The listing builds one solid part. Answer for the finished solid, in the listing's coordinates (mm). Face numbers are marked on the shaded views. Round coordinates to 2 decimals unless told otherwise and drop trailing zeros. Loops run counter-clockwise (first coordinate to the right, second up) from the corner with the lowest first, then second, coordinate; pieces in that order, holes last. Notation, with made-up numbers: (-19.5, 82.5) -> (-12.5, 82.5) arc R32 cw to (-12.5, 115.5) -> close; hole circle Ø5 at (23, -24.75). An arc over 180 degrees is marked (long way). Use a Markdown table: item, result. Add a question column.
Q1. Section A-A on x = -216 is taken. Give the vertices of the cut face in (y, z), then the cut area to 3 significant figures.
Q2. Section D-D on y = 95 is taken. Give the vertices of the cut face in (x, z).
Q3. Section B-B on y = 67 is taken. Give the vertices of the cut face in (x, z).
Q4. Given pin 1 Ø2 at (y, z) = (107.5, -4.5) entering from +X; pin 2 Ø2.5 at (y, z) = (0, 3.5) entering from +X; pin 3 Ø6 at (x, y) = (-211, 23.5) entering from -Z, each flat-ended and moving along its own axis, determine where each tip first touches the part or whether it passes through.
Q5. Section C-C on x = -155 is taken. Give the vertices of the cut face in (y, z).
Q6. For a pull along Y with two mould halves and no side action, classify the marked faces 1, 2 and 3 as released by +Y, released by -Y, zero draft, split by the parting line, or undercut.
Q7. Consider line 1 (Y direction, x = -203, z = 0.75); line 2 (X direction, y = 76, z = 4); line 3 (Y direction, x = -218.5, z = -1). Determine where each line is inside the solid, lowest interval first.
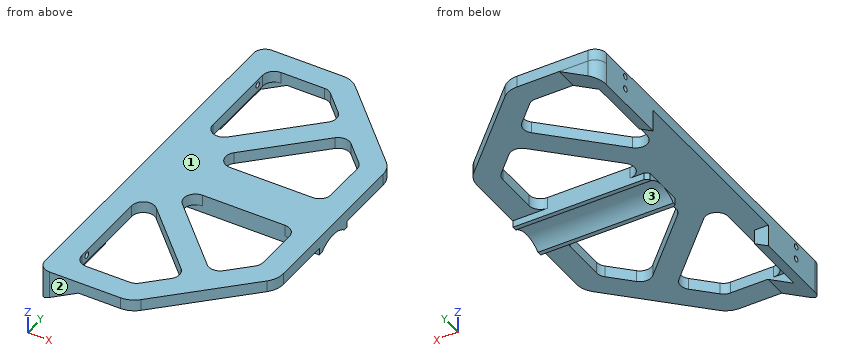
from build123d import *
from build123d.topology import SkipClean

# Parameters (mm, degrees)
RESSALTO_EXTRUS_O2_DEPTH   = 5
CORTE_EXTRUS_O1_DEPTH      = 5
FILETE1_R                  = 10
FILETE2_R                  = 5
ESBO_O7_W                  = 62.928932188
ESBO_O7_H                  = 19.982162149
RESSALTO_EXTRUS_O5_DEPTH   = 5
CORTE_EXTRUS_O2_DEPTH      = 66
FILETE3_R                  = 5
CORTE_EXTRUS_O5_DEPTH      = 35
RESSALTO_EXTRUS_O6_DEPTH   = 159.982162
ESBO_O12_W                 = 11.383352407
ESBO_O12_H                 = 139.982162149
CORTE_EXTRUS_O6_DEPTH      = 10
CORTE_EXTRUS_O7_DEPTH      = 10
CORTE_EXTRUS_O7_DEPTH_BACK = 146.645655307
ESBO_O14_R                 = 1.25
FILETE4_R                  = 5
ESBO_O16_W                 = 30.044355049
ESBO_O16_H                 = 82.897559044
CORTE_EXTRUS_O8_DEPTH      = 262.030945505


with BuildPart() as part:
    # Esboço1 → Ressalto-extrusão2 (new body)
    with BuildSketch(Plane.XY):
        Polygon((-148.870088073, 85.148606513), (-188.870088073, 125.148606513), (-228.870088073, 125.148606513), (-228.870088073, -34.833555636), (-188.870088073, -34.833555636), (-148.870088073, 5.166444364), align=None)
    extrude(amount=RESSALTO_EXTRUS_O2_DEPTH)

    # Esboço4 → Corte-extrusão1 (cut)
    with BuildSketch(Plane(origin=(0, 0, 0), x_dir=(-1, 0, 0), z_dir=(0, 0, -1))):
        Polygon((179.47668979, 101.613072607), (218.870088073, 62.219674325), (218.870088073, 115.148606513), (193.012223696, 115.148606513), align=None)
        Polygon((158.870088073, 55.148606513), (211.799020261, 55.148606513), (172.405621979, 94.542004796), (158.870088073, 81.00647089), align=None)
        Polygon((172.405621979, -4.226953918), (211.799020261, 35.166444364), (158.870088073, 35.166444364), (158.870088073, 9.308579988), align=None)
        Polygon((218.870088073, -24.833555636), (218.870088073, 28.095376552), (179.47668979, -11.29802173), (193.012223696, -24.833555636), align=None)
    extrude(amount=-CORTE_EXTRUS_O1_DEPTH, mode=Mode.SUBTRACT)

    # Filete1
    filete1_edges = [part.edges().sort_by_distance(p)[0] for p in [
        (-188.870088073, 125.148606513, 2.5),
        (-148.870088073, 85.148606513, 2.5),
        (-148.870088073, 5.166444364, 2.5),
        (-188.870088073, -34.833555636, 2.5),
    ]]
    fillet(filete1_edges, radius=FILETE1_R)

    # Filete2
    filete2_edges = [part.edges().sort_by_distance(p)[0] for p in [
        (-218.870088073, 115.148606513, 2.5),
        (-218.870088073, -24.833555636, 2.5),
    ]]
    fillet(filete2_edges, radius=FILETE2_R)

    # Esboço7 → Ressalto-extrusão5 (add)
    with BuildSketch(Plane(origin=(0, 0, 0), x_dir=(-1, 0, 0), z_dir=(0, 0, -1))):
        with Locations((180.334554167, 45.157525439)):
            Rectangle(ESBO_O7_W, ESBO_O7_H)
    extrude(amount=RESSALTO_EXTRUS_O5_DEPTH)

    # Esboço8 → Corte-extrusão2 (cut)
    with BuildSketch(Plane(origin=(-148.870088073, 0, 0), x_dir=(0, 0, -1), z_dir=(1, 0, 0))):
        with BuildLine():
            Line((3.009284908, 37.096966334), (3.009284908, 53.218084544))
            ThreePointArc((3.009284908, 53.218084544), (0, 45.157525439), (3.009284908, 37.096966334))
        make_face()
        with BuildLine():
            Line((5, 55.148606513), (3.009284908, 55.148606513))
            Line((3.009284908, 55.148606513), (3.009284908, 53.218084544))
            ThreePointArc((3.009284908, 53.218084544), (3.95384052, 54.192547406), (5, 55.057020375))
            Line((5, 55.057020375), (5, 55.148606513))
        make_face()
        with BuildLine():
            ThreePointArc((5, 55.057020375), (3.95384052, 54.192547406), (3.009284908, 53.218084544))
            Line((3.009284908, 53.218084544), (3.009284908, 37.096966334))
            ThreePointArc((3.009284908, 37.096966334), (3.95384052, 36.122503472), (5, 35.258030502))
            Line((5, 35.258030502), (5, 55.057020375))
        make_face()
        with BuildLine():
            ThreePointArc((5, 35.258030502), (3.95384052, 36.122503472), (3.009284908, 37.096966334))
            Line((3.009284908, 37.096966334), (3.009284908, 35.166444364))
            Line((3.009284908, 35.166444364), (5, 35.166444364))
            Line((5, 35.166444364), (5, 35.258030502))
        make_face()
    extrude(amount=-CORTE_EXTRUS_O2_DEPTH, mode=Mode.SUBTRACT)

    # Filete3
    filete3_edges = [part.edges().sort_by_distance(p)[0] for p in [
        (-218.870088073, 62.219674325, 2.5),
        (-211.799020261, 55.148606513, 2.5),
        (-211.799020261, 35.166444364, 2.5),
        (-218.870088073, 28.095376552, 2.5),
        (-193.012223696, -24.833555636, 2.5),
        (-179.47668979, -11.29802173, 2.5),
        (-172.405621979, -4.226953918, 2.5),
        (-158.870088073, 9.308579988, 2.5),
        (-158.870088073, 55.148606513, 2.5),
        (-179.47668979, 101.613072607, 2.5),
        (-193.012223696, 115.148606513, 2.5),
        (-158.870088073, 81.00647089, 2.5),
        (-172.405621979, 94.542004796, 2.5),
        (-158.870088073, 35.166444364, 2.5),
    ]]
    fillet(filete3_edges, radius=FILETE3_R)

    # Esboço9 → Corte-extrusão5 (cut)
    # profile 1 of 2: a face of its own
    with BuildSketch(Plane(origin=(0, 0, 0), x_dir=(-1, 0, 0), z_dir=(0, 0, -1))):
        with BuildLine():
            Line((148.870088073, 62.717943557), (158.870088073, 61.569782302))
            Line((158.870088073, 61.569782302), (158.870088073, 78.935403078))
            ThreePointArc((158.870088073, 78.935403078), (159.25069041, 80.84882024), (160.334554167, 82.470936984))
            Line((160.334554167, 82.470936984), (168.870088073, 91.00647089))
            ThreePointArc((168.870088073, 91.00647089), (172.405621979, 92.470936984), (175.941155885, 91.00647089))
            Line((175.941155885, 91.00647089), (203.263486355, 63.684140419))
            ThreePointArc((203.263486355, 63.684140419), (204.725855133, 60.003800568), (203.052854861, 56.414302837))
            ThreePointArc((203.052854861, 56.414302837), (204.549488944, 55.877906361), (205.962201401, 55.148606513))
            Line((205.962201401, 55.148606513), (211.799020261, 55.148606513))
            Line((211.799020261, 55.148606513), (211.799020261, 45.157525439))
            Line((211.799020261, 45.157525439), (211.799020261, 35.166444364))
            Line((211.799020261, 35.166444364), (206.85563775, 35.166444364))
            ThreePointArc((206.85563775, 35.166444364), (205.247649008, 34.173056461), (203.503772873, 33.44412344))
            ThreePointArc((203.503772873, 33.44412344), (204.724845816, 29.990215306), (203.263486355, 26.630910458))
            Line((203.263486355, 26.630910458), (175.941155885, -0.691420012))
            ThreePointArc((175.941155885, -0.691420012), (172.405621979, -2.155886106), (168.870088073, -0.691420012))
            Line((168.870088073, -0.691420012), (160.334554167, 7.844113894))
            ThreePointArc((160.334554167, 7.844113894), (159.25069041, 9.466230638), (158.870088073, 11.3796478))
            Line((158.870088073, 11.3796478), (158.870088073, 26.462519889))
            Line((158.870088073, 26.462519889), (148.870088073, 24.901543221))
            Line((148.870088073, 24.901543221), (148.870088073, 9.308579988))
            ThreePointArc((148.870088073, 9.308579988), (149.631292748, 5.481745664), (151.799020261, 2.237512176))
            Line((151.799020261, 2.237512176), (185.941155885, -31.904623448))
            ThreePointArc((185.941155885, -31.904623448), (189.185389373, -34.072350961), (193.012223696, -34.833555636))
            Line((193.012223696, -34.833555636), (228.870088073, -34.833555636))
            Line((228.870088073, -34.833555636), (228.870088073, 125.148606513))
            Line((228.870088073, 125.148606513), (193.012223696, 125.148606513))
            ThreePointArc((193.012223696, 125.148606513), (189.185389373, 124.387401839), (185.941155885, 122.219674325))
            Line((185.941155885, 122.219674325), (151.799020261, 88.077538702))
            ThreePointArc((151.799020261, 88.077538702), (149.631292748, 84.833305213), (148.870088073, 81.00647089))
            Line((148.870088073, 81.00647089), (148.870088073, 62.717943557))
        make_face()
        with BuildLine():
            ThreePointArc((195.083291508, -24.833555636), (193.169874346, -24.452953298), (191.547757602, -23.369089542))
            Line((191.547757602, -23.369089542), (183.012223696, -14.833555636))
            ThreePointArc((183.012223696, -14.833555636), (181.547757602, -11.29802173), (183.012223696, -7.762487824))
            Line((183.012223696, -7.762487824), (210.334554167, 19.559842647))
            ThreePointArc((210.334554167, 19.559842647), (215.783505235, 20.643706403), (218.870088073, 16.024308741))
            Line((218.870088073, 16.024308741), (218.870088073, -19.833555636))
            ThreePointArc((218.870088073, -19.833555636), (217.405621979, -23.369089542), (213.870088073, -24.833555636))
            Line((213.870088073, -24.833555636), (195.083291508, -24.833555636))
        make_face(mode=Mode.SUBTRACT)
        with BuildLine():
            ThreePointArc((218.870088073, 74.290742137), (215.783505235, 69.671344475), (210.334554167, 70.755208231))
            Line((210.334554167, 70.755208231), (183.012223696, 98.077538702))
            ThreePointArc((183.012223696, 98.077538702), (181.547757602, 101.613072607), (183.012223696, 105.148606513))
            Line((183.012223696, 105.148606513), (191.547757602, 113.684140419))
            ThreePointArc((191.547757602, 113.684140419), (193.169874346, 114.768004176), (195.083291508, 115.148606513))
            Line((195.083291508, 115.148606513), (213.870088073, 115.148606513))
            ThreePointArc((213.870088073, 115.148606513), (217.405621979, 113.684140419), (218.870088073, 110.148606513))
            Line((218.870088073, 110.148606513), (218.870088073, 74.290742137))
        make_face(mode=Mode.SUBTRACT)
    # profile 2 of 2: a face of its own
    with BuildSketch(Plane(origin=(0, 0, 0), x_dir=(-1, 0, 0), z_dir=(0, 0, -1))):
        with BuildLine():
            Line((211.799020261, 55.148606513), (205.962201401, 55.148606513))
            ThreePointArc((205.962201401, 55.148606513), (210.218898447, 50.767748707), (211.771557204, 44.860072713))
            ThreePointArc((211.771557204, 44.860072713), (210.472334539, 39.425629442), (206.85563775, 35.166444364))
            Line((206.85563775, 35.166444364), (211.799020261, 35.166444364))
            Line((211.799020261, 35.166444364), (211.799020261, 45.157525439))
            Line((211.799020261, 45.157525439), (211.799020261, 55.148606513))
        make_face()
    extrude(amount=CORTE_EXTRUS_O5_DEPTH, mode=Mode.SUBTRACT)

    # Esboço10 → Ressalto-extrusão6 (add, through all)
    with SkipClean():  # the faces are left unmerged after this step: merging them gives an invalid solid
        with BuildSketch(Plane.XZ.offset(34.833555636)):
            Polygon((-211.358378387, 0), (-228.870088073, 0), (-228.870088073, -9.667656613), align=None)
        extrude(amount=-RESSALTO_EXTRUS_O6_DEPTH)

    # Esboço12 → Corte-extrusão6 (cut)
    with SkipClean():  # the faces are left unmerged after this step: merging them gives an invalid solid
        with BuildSketch(Plane.XY):
            with Locations((-217.05005459, 45.157525439)):
                Rectangle(ESBO_O12_W, ESBO_O12_H)
        extrude(amount=-CORTE_EXTRUS_O6_DEPTH, mode=Mode.SUBTRACT)

    # Esboço14 → Corte-extrusão7 (cut, two sides: drawn at the far end of the back side and taken through both)
    with SkipClean():  # the faces are left unmerged after this step: merging them gives an invalid solid
        with BuildSketch(Plane(origin=(-222.741730794, 0, 0), x_dir=(0, 0, -1), z_dir=(1, 0, 0)).offset(-CORTE_EXTRUS_O7_DEPTH_BACK)):
            with Locations(Location((2.934607414, 106.56846675, 0), (0, 0, 180))):
                Circle(ESBO_O14_R)
            with Locations(Location((-2.768365458, 106.56846675, 0), (0, 0, 180))):
                Circle(ESBO_O14_R)
            with Locations(Location((-2.768365458, -16.253415872, 0), (0, 0, 180))):
                Circle(ESBO_O14_R)
            with Locations(Location((2.934607414, -16.253415872, 0), (0, 0, 180))):
                Circle(ESBO_O14_R)
        extrude(amount=CORTE_EXTRUS_O7_DEPTH + CORTE_EXTRUS_O7_DEPTH_BACK, mode=Mode.SUBTRACT)

    # Filete4
    filete4_edges = [part.edges().sort_by_distance(p)[0] for p in [
        (-228.870088073, -34.833555636, -4.833828306),
        (-228.870088073, 125.148606364, -4.833828306),
    ]]
    fillet(filete4_edges, radius=FILETE4_R)

    # Esboço16 → Corte-extrusão8 (cut, through all)
    with SkipClean():  # the faces are left unmerged after this step: merging them gives an invalid solid
        with BuildSketch(Plane(origin=(0, 0, 0), x_dir=(-1, 0, 0), z_dir=(0, 0, -1))):
            with Locations((222.741730795, 45.157525439)):
                Rectangle(ESBO_O16_W, ESBO_O16_H)
        extrude(amount=CORTE_EXTRUS_O8_DEPTH, mode=Mode.SUBTRACT)


solid = part.part
Checked values:
| question | item | result |
|---|---|---|
| 1 | outline | (-34.83, -2.56) -> (-24.83, -2.56) -> (-24.83, 0) -> (-24.36, 0) -> (-24.36, 5) -> (-34.83, 5) -> close; (20.55, 0) -> (69.77, 0) -> (69.77, 5) -> (20.55, 5) -> close; (114.67, 0) -> (115.15, 0) -> (115.15, -2.56) -> (125.15, -2.56) -> (125.15, 5) -> (114.67, 5) -> close |
| 1 | area | 402 mm2 |
| 2 | outline | (-228.87, -9.67) -> (-222.74, -6.28) -> (-222.74, 0) -> (-218.87, 0) -> (-218.87, 5) -> (-228.87, 5) -> close; (-186.09, 0) -> (-158.72, 0) -> (-158.72, 5) -> (-186.09, 5) -> close |
| 3 | outline | (-228.87, 0) -> (-199.95, 0) -> (-199.95, 5) -> (-228.87, 5) -> close; (-158.87, 0) -> (-148.87, 0) -> (-148.87, 5) -> (-158.87, 5) -> close |
| 4 | pin 1 | stops at x = -222.74 |
| 4 | pin 2 | stops at x = -152.79 |
| 4 | pin 3 | stops at z = 0 |
| 5 | outline | (-0.96, 0) -> (35.17, 0) -> (35.17, -3.01) -> (37.1, -3.01) arc R12.3 cw to (53.22, -3.01) -> (55.15, -3.01) -> (55.15, 0) -> (91.28, 0) -> (91.28, 5) -> (-0.96, 5) -> close |
| 6 | face 1 | zero draft |
| 6 | face 2 | released by -Y |
| 6 | face 3 | undercut |
| 7 | line 1 | y = -34.83 to -24.83, 12.23 to 26.37, 33.95 to 56.37, 63.95 to 78.09, 115.15 to 125.15 |
| 7 | line 2 | x = -228.87 to -218.87, -205.09 to -190.95, -158.87 to -148.87 |
| 7 | line 3 | y = -34.83 to -24.83, 115.15 to 125.15 |
